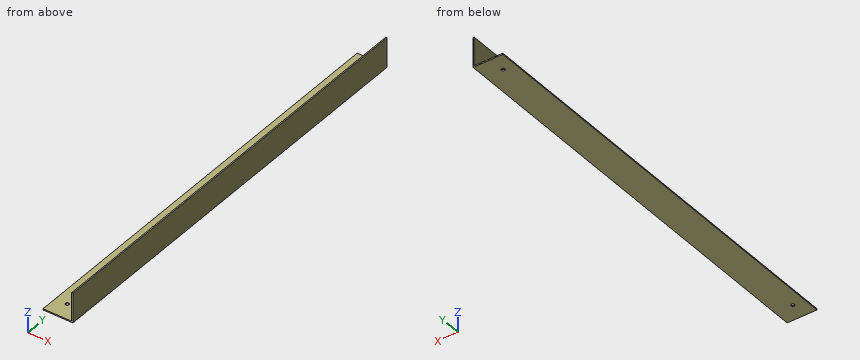
```python
from build123d import *

# Parameters (mm, degrees)
CROQUIS1_W              = 24
CROQUIS1_H              = 360
CROQUIS1_R              = 1.5
SALIENTE_EXTRUIR1_DEPTH = 1
CROQUIS2_W              = 1
CROQUIS2_H              = 360
SALIENTE_EXTRUIR2_DEPTH = 25


with BuildPart() as part:
    # Croquis1 → Saliente-Extruir1 (new body)
    with BuildSketch(Plane.XY):
        with Locations((-41.401725042, -153.514805415)):
            Rectangle(CROQUIS1_W, CROQUIS1_H)
        with Locations((-43.401725042, 12.485194585)):
            Circle(CROQUIS1_R, mode=Mode.SUBTRACT)
        with Locations((-43.401725042, -319.514805415)):
            Circle(CROQUIS1_R, mode=Mode.SUBTRACT)
    extrude(amount=SALIENTE_EXTRUIR1_DEPTH)

    # Croquis2 → Saliente-Extruir2 (add)
    with BuildSketch(Plane.XY):
        with Locations((-28.901725042, -153.514805415)):
            Rectangle(CROQUIS2_W, CROQUIS2_H)
    extrude(amount=SALIENTE_EXTRUIR2_DEPTH)


solid = part.part
```
Verification items for the finished model (mm, model axes). Round coordinates to 2 decimals unless told otherwise and drop trailing zeros. Order: outer loops, then holes, each group sorted by start corner. A loop starts at its lowest first (then second) coordinate and runs counter-clockwise, first axis right, second up. Notation, with made-up numbers: (36.25, 2) - (60.25, 2) arc R28 ccw to (60.25, 27) - close; hole circle Ø7 at (71.25, 7.25). An arc over 180 degrees is marked (long way). Use CSV: the item, a comma, the result in double quotes. Start each with the question number.
1) Section check B-B, the plane x = -32.75. Record the cut outline in (y, z), plus the area to 3 significant figures.
2) Thickness scan on L1, parallel to X at y = -19.5, z = 14; L2, parallel to Z at x = -37.75, y = -226. Record the ranges inside material, lowest first.
3) Go/stop test with flat-tipped pins: P1, Ø1, axis at x = -50, y = -268.5, coming from the +Z side; P2, Ø4, axis at y = -118, z = 14.5, coming from the -X side; P3, Ø5, axis at x = -49.5, z = 5, coming from the -Y side. Record where each tip stops, or that it passes through.
4) Section check A-A, the plane y = -258.5. Record the cut outline in (x, z).
5) Section check C-C, the plane z = 22. Record the cut outline in (x, y).
Answers:
1,outline,"(-333.51, 0) - (26.49, 0) - (26.49, 1) - (-333.51, 1) - close"
1,area,"360 mm²"
2,L1,"x = -29.4 to -28.4"
2,L2,"z = 0 to 1"
3,P1,"stops at z = 1"
3,P2,"stops at x = -29.4"
3,P3,"passes through"
4,outline,"(-53.4, 0) - (-28.4, 0) - (-28.4, 25) - (-29.4, 25) - (-29.4, 1) - (-53.4, 1) - close"
5,outline,"(-29.4, -333.51) - (-28.4, -333.51) - (-28.4, 26.49) - (-29.4, 26.49) - close"
